from build123d import *

# Parameters (mm, degrees)
F0_W      = 24
F0_H      = 28
F0_W_2    = 15
F0_H_2    = 20
F1_DEPTH  = 1.5
F2_W      = 24
F2_H      = 28
F2_W_2    = 20
F2_H_2    = 24
F3_DEPTH  = 30
F4_R      = 2
F5_DEPTH  = 1
F6_R      = 2
F7_DEPTH  = 1
F8_R      = 0.99999
F9_W      = 12
F9_H      = 3
F10_DEPTH = 2


# Not quite as in the source:
# - a fillet or chamfer is up to 0.001 mm smaller than in the source, because OpenCascade refuses the exact size


with BuildPart() as f1:
    # F0 (on Top) → F1 (new body)
    with BuildSketch(Plane.XY):
        Rectangle(F0_W, F0_H)
        Rectangle(F0_W_2, F0_H_2, mode=Mode.SUBTRACT)
    extrude(amount=F1_DEPTH)

    # F2 (on face) → F3 (join)
    with BuildSketch(Plane.XY.offset(1.5)):
        Rectangle(F2_W, F2_H)
        Rectangle(F2_W_2, F2_H_2, mode=Mode.SUBTRACT)
    extrude(amount=F3_DEPTH)

    # F4 (on face) → F5 (cut)
    with BuildSketch(Plane.YZ.offset(-10)):
        with Locations((-4, 28)):
            Circle(F4_R)
        with Locations((4, 28)):
            Circle(F4_R)
    extrude(amount=-F5_DEPTH, mode=Mode.SUBTRACT)

    # F6 (on face) → F7 (cut)
    with BuildSketch(Plane(origin=(10, 0, 0), x_dir=(0, -1, 0), z_dir=(-1, 0, 0))):
        with Locations((4, 28)):
            Circle(F6_R)
        with Locations((-4, 28)):
            Circle(F6_R)
    extrude(amount=-F7_DEPTH, mode=Mode.SUBTRACT)

    # F8 (radius 1 in the source; OpenCascade refuses exactly that, so slightly less here)
    f8_edges = [f1.edges().sort_by_distance(p)[0] for p in [
        (11, -2, 28),
        (11, 6, 28),
        (-11, -6, 28),
        (-11, 2, 28),
    ]]
    fillet(f8_edges, radius=F8_R)

    # F9 (on face) → F10 (cut, through all)
    with BuildSketch(Plane(origin=(0, 14, 0), x_dir=(-1, 0, 0), z_dir=(0, 1, 0))):
        with Locations((0, 28)):
            Rectangle(F9_W, F9_H)
    extrude(amount=-F10_DEPTH, mode=Mode.SUBTRACT)


solid = f1.part
Here's how the part is built. I have some questions about the finished solid (model axes, mm). A direction names the side the tool comes from. Round coordinates to 2 decimals unless told otherwise and drop trailing zeros. Loops run counter-clockwise (first coordinate to the right, second up) from the corner with the lowest first, then second, coordinate; pieces in that order, holes last. Notation, with made-up numbers: (-10, 50) - (25, 50) arc R26 ccw to (25, 82) - close; hole circle Ø10 at (47.5, -28). An arc over 180 degrees is marked (long way). One line per question, with ' | ' between items. Start each with the question number.
Q1. I want a section at D-D (z = 4.5). Write out the boundary of the cut face in (x, y), then the cut area to 3 significant figures.
Q2. I want a section at C-C (x = 5). Write out the boundary of the cut face in (y, z), then the cut area to 3 significant figures.
Q3. We'd pull the mould along Y, two halves only. Please class faces 6 (the flat face through (0, -14, 16)), 7 (the flat face through (-10, 0, 16)), 8 (the flat face through (0, 12, 16)), 9 (the flat face through (6, 13, 28)): +Y half, -Y half, draft (parallel to the pull), parting line (faces both ways), or undercut.
Q4. I want a section at A-A (x = -6.75). Write out the boundary of the cut face in (y, z).
Q5. For faces 1 (the flat face through (-12, 0, 16)), 2 (the flat face through (11, 4, 28)), 3 (the flat face through (-7.5, 0, 1)), 4 (the flat face through (-9, 0, 1.5)), 5 (the flat face through (0, 13, 26.5)), which set-ups out of +Z, -Z, +X, -X, +Y, -Y let a thin tool reach every point of the face, with its end or its side?
Q6. Please list where these lines run through material, in increasing order: line 1 (X direction, y = -2, z = 12.5); line 2 (Y direction, x = 4.5, z = 5.5); line 3 (Z direction, x = 10.05, y = -4). Write a range as [from, to].
Q7. I want a section at B-B (y = 8.75). Write out the boundary of the cut face in (x, z), then the cut area to 4 significant figures.
Response values:
1) outline: (-12, -14) - (12, -14) - (12, 14) - (-12, 14) - close; hole (-10, -12) - (10, -12) - (10, 12) - (-10, 12) - close | area: 192 mm²
2) outline: (-14, 0) - (-10, 0) - (-10, 1.5) - (-12, 1.5) - (-12, 31.5) - (-14, 31.5) - close; (10, 0) - (14, 0) - (14, 26.5) - (12, 26.5) - (12, 1.5) - (10, 1.5) - close; (12, 29.5) - (14, 29.5) - (14, 31.5) - (12, 31.5) - close | area: 126 mm²
3) face 6: -Y half | face 7: undercut | face 8: undercut | face 9: draft
4) outline: (-14, 0) - (-10, 0) - (-10, 1.5) - (-12, 1.5) - (-12, 31.5) - (-14, 31.5) - close; (10, 0) - (14, 0) - (14, 31.5) - (12, 31.5) - (12, 1.5) - (10, 1.5) - close
5) face 1: +Z, -Z, -X, +Y, -Y | face 2: none | face 3: +Z, -Z | face 4: +Z | face 5: +Y
6) line 1: x = [-12, -10], [10, 12] | line 2: y = [-14, -12], [12, 14] | line 3: z = [0, 26], [30, 31.5]
7) outline: (-12, 0) - (-7.5, 0) - (-7.5, 1.5) - (-10, 1.5) - (-10, 31.5) - (-12, 31.5) - close; (7.5, 0) - (12, 0) - (12, 31.5) - (10, 31.5) - (10, 1.5) - (7.5, 1.5) - close | area: 133.5 mm²
